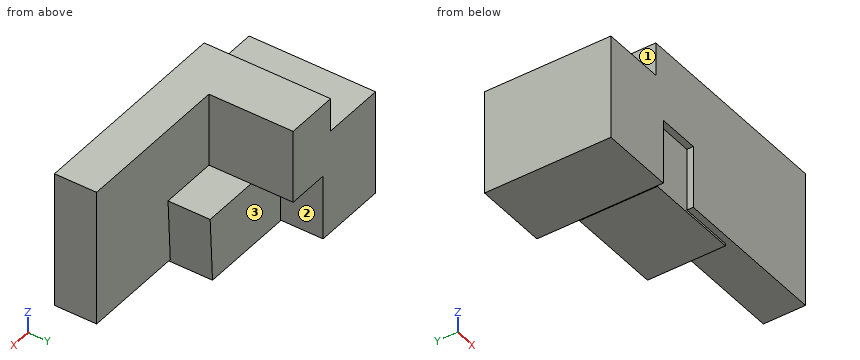
```python
from build123d import *

# Parameters (mm, degrees)
SKETCH1_W           = 190.5
SKETCH1_H           = 165.1
BOSS_EXTRUDE1_DEPTH = 50.8
SKETCH2_W           = 88.9
SKETCH2_H           = 152.4
BOSS_EXTRUDE2_DEPTH = 63.5
BOSS_EXTRUDE3_DEPTH = 152.4
BOSS_EXTRUDE4_DEPTH = 93.98


with BuildPart() as part:
    # Sketch1 → Boss-Extrude1 (new body)
    with BuildSketch(Plane(origin=(0, 0, 0), x_dir=(1, 0, 0), z_dir=(0, 1, 0))):
        Rectangle(SKETCH1_W, SKETCH1_H)
    extrude(amount=BOSS_EXTRUDE1_DEPTH)

    # Sketch2 → Boss-Extrude2 (add)
    with BuildSketch(Plane.ZY.offset(95.25)):
        with Locations((38.1, 76.2)):
            Rectangle(SKETCH2_W, SKETCH2_H)
    extrude(amount=BOSS_EXTRUDE2_DEPTH)

    # Sketch3 → Boss-Extrude3 (add)
    with BuildSketch(Plane(origin=(0, 152.4, 0), x_dir=(1, 0, 0), z_dir=(0, 1, 0))):
        Polygon((-158.75, 6.35), (-146.05, 6.35), (-146.05, 85.09), (-235.014810015, 85.09), (-235.014810015, -41.91), (-158.75, -41.91), align=None)
    extrude(amount=-BOSS_EXTRUDE3_DEPTH)

    # Sketch9 → Boss-Extrude4 (add)
    with BuildSketch(Plane(origin=(0, 101.6, 0), x_dir=(1, 0, 0), z_dir=(0, 1, 0))):
        Polygon((-145.392235631, 6.475919558), (-145.392235631, 85.217024974), (-29.908989465, 85.217024974), (-25.920545989, 6.475919558), align=None)
    extrude(amount=-BOSS_EXTRUDE4_DEPTH)


solid = part.part
```
Here's how the part is built. I have some questions about the finished solid (model axes, mm). Face numbers are marked on the shaded views. A direction names the side the tool comes from. Round coordinates to 2 decimals unless told otherwise and drop trailing zeros. Write each loop counter-clockwise with the first axis right and the second up, starting at its lowest first coordinate (ties: lowest second). Pieces come first, ordered by that corner, then holes.
Q1. Please list where these lines run through material, in increasing order: probe 1 along X at (y, z) = (24, -63); probe 2 along Z at (x, y) = (-83, 59); probe 3 along Y at (x, z) = (-27, 19.5).
Q2. If we section it at B-B on z = -47.5: Write out the boundary of the cut face in (x, y).
Q3. If we section it at D-D on z = 57.5: Write out the boundary of the cut face in (x, y), plus the area to 3 significant figures.
Q4. If we section it at A-A on x = -99: Write out the boundary of the cut face in (y, z), plus the area to 3 significant figures.
Q5. Will these pins go through, and if not, where does the flat tip stop? P1, Ø23.5, axis at x = -108, z = -28.5, coming from the +Y side; P2, Ø15, axis at x = 17.5, y = 28, coming from the -Z side; P3, Ø4, axis at x = -164.5, y = 115.5, coming from the -Z side; P4, Ø2, axis at x = 25.5, z = -9.5, coming from the -Y side.
Q6. Which directions (+Z, -Z, +X, -X, +Y, -Y) give clear straight access to the entire face, cutting with the end or side of a thin tool? Please do the marked faces 1, 2 and 3.
Q7. If we section it at C-C on y = 135: Write out the boundary of the cut face in (x, z).
Answer below:
1. probe 1: x = -235.01 to -146.05, -145.39 to 95.25
1. probe 2: z = -85.22 to -6.48
1. probe 3: y = 0 to 50.8
2. outline: (-235.01, 0) - (-146.05, 0) - (-146.05, 152.4) - (-235.01, 152.4) - close; (-145.39, 7.62) - (-95.25, 7.62) - (-95.25, 0) - (95.25, 0) - (95.25, 50.8) - (-28, 50.8) - (-28, 101.6) - (-145.39, 101.6) - close
3. outline: (-158.75, 0) - (95.25, 0) - (95.25, 50.8) - (-95.25, 50.8) - (-95.25, 152.4) - (-158.75, 152.4) - close
3. area: 19,400 mm2
4. outline: (0, -6.35) - (152.4, -6.35) - (152.4, 82.55) - (0, 82.55) - close; (7.62, -85.22) - (101.6, -85.22) - (101.6, -6.48) - (7.62, -6.48) - close
4. area: 20,900 mm2
5. P1: stops at y = 101.6
5. P2: stops at z = -82.55
5. P3: stops at z = -85.09
5. P4: stops at y = 0
6. face 1: +Z, -X, +Y, -Y
6. face 2: -Z, +Y, -Y
6. face 3: -Z, +X, +Y
7. outline: (-235.01, -85.09) - (-146.05, -85.09) - (-146.05, -6.35) - (-95.25, -6.35) - (-95.25, 82.55) - (-158.75, 82.55) - (-158.75, 41.91) - (-235.01, 41.91) - close
